The figure shows three views and two pictorial views of one solid part (mm, origin at its lowest corner). Answer the questions. Coordinates: 2 decimals unless noted, no trailing zeros. Loops run counter-clockwise (first coordinate to the right, second up) from the corner with the lowest first, then second, coordinate; pieces in that order, holes last.
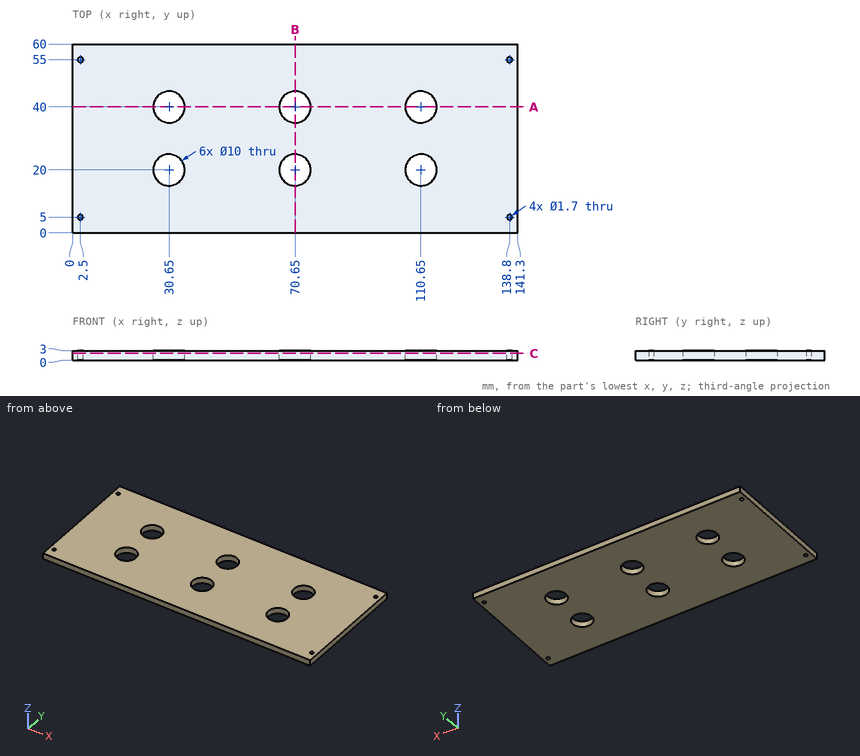
1. A cutting plane is placed at C-C, the plane z = 2.2. Count the separate pieces of the cut face and the enclosed holes in it, then the cut area to 3 significant figures.
2. Straight lines are drawn through the part: probe 1 along Y at (x, z) = (30.65, 0.65); probe 2 along Y at (x, z) = (138.8, 2.05); probe 3 along X at (y, z) = (41.5, 1). For each, find the intervals that lie inside material, in ascending order.
3. A cutting plane is placed at B-B, the plane x = 70.65. Give the vertices of the cut face in (y, z), then the cut area to 3 significant figures.
4. A cutting plane is placed at A-A, the plane y = 40. Give the vertices of the cut face in (x, z).
Answers below:
1. separate pieces: 1
1. enclosed holes: 10
1. area: 8,000 mm2
2. probe 1: y = 0 to 15, 25 to 35, 45 to 60
2. probe 2: y = 0 to 4.15, 5.85 to 54.15, 55.85 to 60
2. probe 3: x = 0 to 25.88, 35.42 to 65.88, 75.42 to 105.88, 115.42 to 141.3
3. outline: (0, 0) - (15, 0) - (15, 3) - (0, 3) - close; (25, 0) - (35, 0) - (35, 3) - (25, 3) - close; (45, 0) - (60, 0) - (60, 3) - (45, 3) - close
3. area: 120 mm2
4. outline: (0, 0) - (25.65, 0) - (25.65, 3) - (0, 3) - close; (35.65, 0) - (65.65, 0) - (65.65, 3) - (35.65, 3) - close; (75.65, 0) - (105.65, 0) - (105.65, 3) - (75.65, 3) - close; (115.65, 0) - (141.3, 0) - (141.3, 3) - (115.65, 3) - close
